Source: CAD feature listing. Evaluate the final solid. Frame: model axes, mm. A direction names the side the tool comes from. Give positions to 0.01 mm unless a question says otherwise; leave off trailing zeros. Order: outer loops, then holes, each group sorted by start corner. A loop starts at its lowest first (then second) coordinate and runs counter-clockwise, first axis right, second up. Notation, with made-up numbers: M 24.25,4 L 32.25,4 A25 cw 32.25,34 Z; hole C 52.25,16 d6. An arc over 180 degrees is marked long. Answer as a JSON object with one key per item and string values. Group by question number.
1. Section query B-B (z = 11). Output: boundary loops of the cut face in (x, y) (3 decimals), plus the area to 3 significant figures.
2. Material intervals for L1, parallel to Z at x = -22, y = 1.25 (3 decimals); L2, parallel to X at y = 3.45, z = 4 (3 decimals); L3, parallel to Z at x = -8, y = 3.35, sorted ascending. Write a range as [from, to].
3. Pin query (flat end, axial travel): P1, Ø3, axis at x = -37.22, z = 24.12, coming from the -Y side; P2, Ø2.5, axis at x = 37.22, z = 24.12, coming from the +Y side. Return the tip coordinate at first contact, or that it passes through.
4. Section query A-A (x = 9). Output: boundary loops of the cut face in (y, z).
5. Pull-direction query (Z, two-part tool) for faces 6 (the flat face through (-1, 2, -35)), 7 (the flat face through (-54, 2, 0)), 8 (the flat face through (35.83, 1.48, 15.74)); classes: +Z half, -Z half, draft (parallel to the pull), parting line (faces both ways), or undercut.
6. Set-up query: faces 1 (the flat face through (54, 2, 0)), 2 (the flat face through (33, 5, -8)), 3 (the flat face through (19, 3, -21.125)), 4 (the flat face through (-14.866, 4.507, -28.995)), 5 (the cylindrical face through (-36.89, 1.48, -32.24)). Return all of +Z, -Z, +X, -X, +Y, -Y with unobstructed straight access to the full face (end or side cutting, diameter ignored); none if empty.
from build123d import *

# Parameters (mm, degrees)
SCHIZZO1_W                   = 108
SCHIZZO1_H                   = 70
SCHIZZO1_R                   = 8.125
ESTRUSIONE_ESTRUSIONE2_DEPTH = 5
TAGLIO_ESTRUSIONE4_DEPTH     = 1
SCHIZZO8_R                   = 1.88
TAGLIO_ESTRUSIONE5_DEPTH     = 95
SCHIZZO9_W                   = 54
SCHIZZO9_H                   = 42
TAGLIO_ESTRUSIONE6_DEPTH     = 10
SCHIZZO10_W                  = 22.988764944
SCHIZZO10_H                  = 46.310438252
TAGLIO_ESTRUSIONE7_DEPTH     = 10
SCHIZZO11_W                  = 54.25
SCHIZZO11_H                  = 42.25
TAGLIO_ESTRUSIONE8_DEPTH     = 10
SCHIZZO14_R                  = 8.125
ESTRUSIONE_ESTRUSIONE3_DEPTH = 2
SCHIZZO15_R                  = 8.125
ESTRUSIONE_ESTRUSIONE4_DEPTH = 2
TAGLIO_ESTRUSIONE10_DEPTH    = 3
SCHIZZO17_R                  = 1
TAGLIO_ESTRUSIONE11_DEPTH    = 3


with BuildPart() as part:
    # Schizzo1 → Estrusione-Estrusione2 (new body)
    with BuildSketch(Plane(origin=(0, 0, 0), x_dir=(1, 0, 0), z_dir=(0, 1, 0))):
        Rectangle(SCHIZZO1_W, SCHIZZO1_H)
        with Locations((-37.216940269, -24.122090915)):
            Circle(SCHIZZO1_R, mode=Mode.SUBTRACT)
        with Locations((-37.216940269, 24.122090915)):
            Circle(SCHIZZO1_R, mode=Mode.SUBTRACT)
        with Locations((37.216940269, 24.122090915)):
            Circle(SCHIZZO1_R, mode=Mode.SUBTRACT)
        with Locations((37.216940269, -24.122090915)):
            Circle(SCHIZZO1_R, mode=Mode.SUBTRACT)
        with BuildLine():
            Line((16.970562748, 21), (-16.970562748, 21))
            ThreePointArc((-16.970562748, 21), (-27, 0), (-16.970562748, -21))
            Line((-16.970562748, -21), (16.970562748, -21))
            ThreePointArc((16.970562748, -21), (27, 0), (16.970562748, 21))
        make_face(mode=Mode.SUBTRACT)
    extrude(amount=ESTRUSIONE_ESTRUSIONE2_DEPTH)

    # Schizzo5 → Taglio-Estrusione4 (cut)
    with BuildSketch(Plane(origin=(0, 5, 0), x_dir=(1, 0, 0), z_dir=(0, 1, 0))):
        Polygon((-22.093333333, 35), (18.323333333, -35), (22.083333333, -35), (-18.333333333, 35), align=None)
    extrude(amount=-TAGLIO_ESTRUSIONE4_DEPTH, mode=Mode.SUBTRACT)

    # Schizzo8 → Taglio-Estrusione5 (cut, along a direction that is not the sketch's normal)
    with BuildSketch(Plane.XY.offset(35)):
        with Locations((20.203333333, 4)):
            Circle(SCHIZZO8_R)
    extrude(amount=-TAGLIO_ESTRUSIONE5_DEPTH, dir=(0.500019929, 0, 0.866013898), mode=Mode.SUBTRACT)

    # Schizzo9 → Taglio-Estrusione6 (cut)
    with BuildSketch(Plane(origin=(0, 5, 0), x_dir=(1, 0, 0), z_dir=(0, 1, 0))):
        Rectangle(SCHIZZO9_W, SCHIZZO9_H)
    extrude(amount=-TAGLIO_ESTRUSIONE6_DEPTH, mode=Mode.SUBTRACT)

    # Schizzo10 → Taglio-Estrusione7 (cut)
    with BuildSketch(Plane(origin=(0, 5, 0), x_dir=(1, 0, 0), z_dir=(0, 1, 0))):
        Rectangle(SCHIZZO10_W, SCHIZZO10_H)
    extrude(amount=-TAGLIO_ESTRUSIONE7_DEPTH, mode=Mode.SUBTRACT)

    # Schizzo11 → Taglio-Estrusione8 (cut)
    with BuildSketch(Plane(origin=(0, 5, 0), x_dir=(1, 0, 0), z_dir=(0, 1, 0))):
        Rectangle(SCHIZZO11_W, SCHIZZO11_H)
    extrude(amount=-TAGLIO_ESTRUSIONE8_DEPTH, mode=Mode.SUBTRACT)

    # Schizzo14 → Estrusione-Estrusione3 (add)
    with BuildSketch(Plane(origin=(0, 5, 0), x_dir=(1, 0, 0), z_dir=(0, 1, 0))):
        with Locations((37.216940269, 24.122090915)):
            Circle(SCHIZZO14_R)
        with Locations((37.216940269, -24.122090915)):
            Circle(SCHIZZO14_R)
    extrude(amount=-ESTRUSIONE_ESTRUSIONE3_DEPTH)

    # Schizzo15 → Estrusione-Estrusione4 (add)
    with BuildSketch(Plane(origin=(0, 5, 0), x_dir=(1, 0, 0), z_dir=(0, 1, 0))):
        with Locations((-37.216940269, 24.122090915)):
            Circle(SCHIZZO15_R)
        with Locations((-37.216940269, -24.122090915)):
            Circle(SCHIZZO15_R)
    extrude(amount=-ESTRUSIONE_ESTRUSIONE4_DEPTH)

    # Schizzo16 → Taglio-Estrusione10 (cut)
    with BuildSketch(Plane.XZ):
        Polygon((-40.023183309, 16.497090915), (-34.410697229, 16.497090915), (-37.216940269, 14.997090915), align=None)
        Polygon((-40.023183309, -16.622090915), (-34.410697229, -16.622090915), (-37.216940269, -15.122090915), align=None)
        Polygon((34.410697229, 16.497090915), (40.023183309, 16.497090915), (37.216940269, 14.997090915), align=None)
        Polygon((34.091940269, -16.622090915), (37.216940269, -15.122090915), (40.341940269, -16.622090915), align=None)
    extrude(amount=-TAGLIO_ESTRUSIONE10_DEPTH, mode=Mode.SUBTRACT)

    # Schizzo17 → Taglio-Estrusione11 (cut)
    with BuildSketch(Plane.XZ.offset(-3)):
        with Locations((-37.216940269, 24.122090915)):
            Circle(SCHIZZO17_R)
        with Locations((37.216940269, 24.122090915)):
            Circle(SCHIZZO17_R)
        with Locations((37.216940269, -24.122090915)):
            Circle(SCHIZZO17_R)
        with Locations((-37.216940269, -24.122090915)):
            Circle(SCHIZZO17_R)
    extrude(amount=-TAGLIO_ESTRUSIONE11_DEPTH, mode=Mode.SUBTRACT)


solid = part.part
Answer sheet:
{
 "1": {"outline": "M -54,0 L -27.125,0 L -27.125,5 L -54,5 Z; M 27.125,0 L 54,0 L 54,5 L 27.125,5 Z", "area": "269 mm^2"},
 "2": {"L1": "[-35, -21.125], [21.125, 35]", "L2": "[-54, -27.125], [27.125, 54]", "L3": "[-35, -23.16], [23.16, 35]"},
 "3": {"P1": "y = 3", "P2": "y = 5"},
 "4": {"outline": "M 0,-35 L 5,-35 L 5,-23.16 L 0,-23.16 Z; M 0,23.16 L 5,23.16 L 5,35 L 0,35 Z"},
 "5": {"face 6": "-Z half", "face 7": "draft", "face 8": "undercut"},
 "6": {"face 1": "+Z, -Z, +X, +Y, -Y", "face 2": "+Z, -Z, +X, -X, +Y", "face 3": "+Y, -Y", "face 4": "+Y", "face 5": "-Y"}
}
